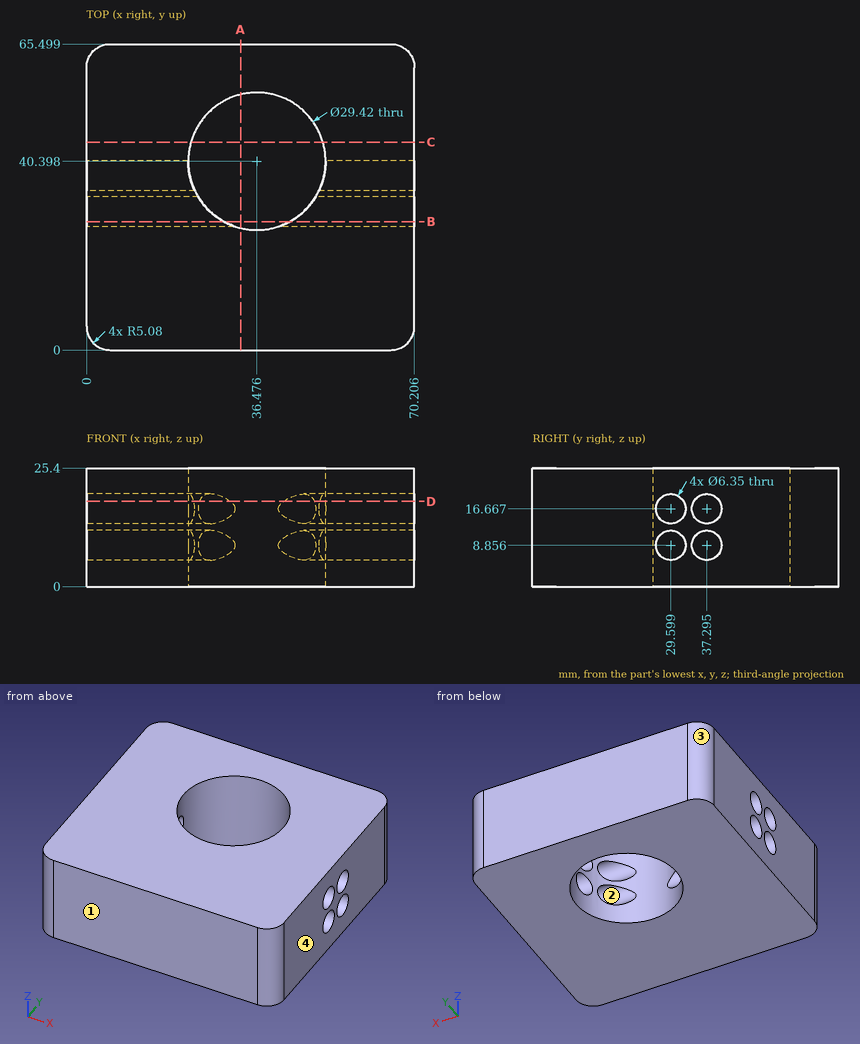
Could you check a few things on this drawing? It's one solid part, dimensions in mm from its lowest x, y, z. Coordinates: 2 decimals unless noted, no trailing zeros. Loops run counter-clockwise (first coordinate to the right, second up) from the corner with the lowest first, then second, coordinate; pieces in that order, holes last. Notation, with made-up numbers: (43, 37.25) - (68, 37.25) arc R29 ccw to (68, 64.25) - close; hole circle Ø8 at (64.25, -40). An arc over 180 degrees is marked (long way). Return JSON: item names as keys, results as strings. Group by question number.
Item 1: If we section it at D-D on z = 18.25: Write out the boundary of the cut face in (x, y) (1 decimal).
Item 2: Will this pin go through, and if not, where does the flat tip stop? P1, Ø4, axis at y = 37.3, z = 16.67, coming from the +X side.
Item 3: We'd pull the mould along Y, two halves only. Please class the marked faces 1, 2, 3 and 4: +Y half, -Y half, draft (parallel to the pull), parting line (faces both ways), or undercut.
Item 4: If we section it at C-C on y = 44.5: Write out the boundary of the cut face in (x, z) (1 decimal), and give its area (3 significant figures).
Item 5: If we section it at A-A on x = 33: Write out the boundary of the cut face in (y, z).
Item 6: If we section it at B-B on y = 27.5: State how many separate pieces and enclosed holes the cut face has.
Item 7: I need wall thicknesses on line 1 (Y direction, x = 11.5, z = 8) (1 decimal); line 2 (Y direction, x = 19.5, z = 11) (1 decimal); line 3 (Y direction, x = 37, z = 2.5). Which ranges of each line are inside material? Lowest first, please. Write a range as from..to.
Calculated:
{
 "1": {"outline": "(0, 5.1) arc R5.1 ccw to (5.1, 0) - (65.1, 0) arc R5.1 ccw to (70.2, 5.1) - (70.2, 26.8) - (42.2, 26.8) arc R14.7 cw to (30.8, 26.8) - (0, 26.8) - close; (0, 32.4) - (24.2, 32.4) arc R14.7 cw to (23, 34.5) - (0, 34.5) - close; (0, 40) - (21.8, 40) arc R14.7 cw (long way) to (51.2, 40) - (70.2, 40) - (70.2, 60.4) arc R5.1 ccw to (65.1, 65.5) - (5.1, 65.5) arc R5.1 ccw to (0, 60.4) - close; (48.8, 32.4) - (70.2, 32.4) - (70.2, 34.5) - (50, 34.5) arc R14.7 cw to start"},
 "2": {"P1": "passes through"},
 "3": {"face 1": "-Y half", "face 2": "undercut", "face 3": "+Y half", "face 4": "draft"},
 "4": {"outline": "(0, 0) - (22.3, 0) - (22.3, 25.4) - (0, 25.4) - close; (50.6, 0) - (70.2, 0) - (70.2, 25.4) - (50.6, 25.4) - close", "area": "1,070 mm^2"},
 "5": {"outline": "(0, 0) - (26.1, 0) - (26.1, 25.4) - (0, 25.4) - close; (54.69, 0) - (65.5, 0) - (65.5, 25.4) - (54.69, 25.4) - close"},
 "6": {"separate pieces": "6", "enclosed holes": "0"},
 "7": {"line 1": "y = 0..26.5, 32.7..34.2, 40.4..65.5", "line 2": "y = 0..27.3, 31.9..35, 39.6..65.5", "line 3": "y = 0..25.7, 55.1..65.5"}
}
